The listing builds one solid part. Answer for the finished solid, in the listing's coordinates (mm). A direction names the side the tool comes from. Give positions to 0.01 mm unless a question says otherwise; leave off trailing zeros. Order: outer loops, then holes, each group sorted by start corner. A loop starts at its lowest first (then second) coordinate and runs counter-clockwise, first axis right, second up.
```python
from build123d import *

# Parameters (mm, degrees)
BOSS_EXTRUDE1_DEPTH = 5
FILLET1_R           = 8
BOSS_EXTRUDE2_DEPTH = 35
CUT_EXTRUDE1_DEPTH  = 40
CUT_EXTRUDE2_DEPTH  = 5
SKETCH9_W           = 9.5
SKETCH9_H           = 40
BOSS_EXTRUDE3_DEPTH = 3
SKETCH10_R          = 1.6
SKETCH10_W          = 6
SKETCH10_H          = 10
CUT_EXTRUDE3_DEPTH  = 3
SKETCH11_W          = 9.5
SKETCH11_H          = 4
BOSS_EXTRUDE4_DEPTH = 40
SKETCH13_W          = 25
SKETCH13_H          = 5
BOSS_EXTRUDE5_DEPTH = 15
SKETCH15_R          = 1.6
CUT_EXTRUDE4_DEPTH  = 5
CUT_EXTRUDE5_DEPTH  = 5
SKETCH17_W          = 17
SKETCH17_H          = 5
BOSS_EXTRUDE6_DEPTH = 9
SKETCH18_R          = 1.6
CUT_EXTRUDE6_DEPTH  = 5
CUT_EXTRUDE8_DEPTH  = 5


with BuildPart() as part:
    # Sketch1 → Boss-Extrude1 (new body)
    with BuildSketch(Plane(origin=(0, 0, 0), x_dir=(1, 0, 0), z_dir=(0, 1, 0))):
        Polygon((-75.055534995, 0), (-37.527767497, -65), (37.527767497, -65), (75.055534995, 0), (37.527767497, 65), (-37.527767497, 65), align=None)
    extrude(amount=BOSS_EXTRUDE1_DEPTH)

    # Fillet1
    fillet1_edges = [part.edges().sort_by_distance(p)[0] for p in [
        (-37.527767497, 2.5, -65),
        (37.527767497, 2.5, -65),
        (75.055534995, 2.5, 0),
        (37.527767497, 2.5, 65),
        (-37.527767497, 2.5, 65),
        (-75.055534995, 2.5, 0),
    ]]
    fillet(fillet1_edges, radius=FILLET1_R)

    # Sketch3 → Boss-Extrude2 (add)
    with BuildSketch(Plane(origin=(0, 5, 0), x_dir=(1, 0, 0), z_dir=(0, 1, 0))):
        with BuildLine():
            Line((-25, 65), (25, 65))
            ThreePointArc((25, 65), (30.656854249, 62.656854249), (33, 57))
            Line((33, 57), (33, -57))
            ThreePointArc((33, -57), (30.656854249, -62.656854249), (25, -65))
            Line((25, -65), (-25, -65))
            ThreePointArc((-25, -65), (-30.656854249, -62.656854249), (-33, -57))
            Line((-33, -57), (-33, 57))
            ThreePointArc((-33, 57), (-30.656854249, 62.656854249), (-25, 65))
        make_face()
    extrude(amount=BOSS_EXTRUDE2_DEPTH)

    # Sketch4 → Cut-Extrude1 (cut)
    with BuildSketch(Plane(origin=(0, 40, 0), x_dir=(1, 0, 0), z_dir=(0, 1, 0))):
        Polygon((-28, 57), (-25, 60), (25, 60), (28, 57), (28, -57), (25, -60), (-25, -60), (-28, -57), align=None)
    extrude(amount=-CUT_EXTRUDE1_DEPTH, mode=Mode.SUBTRACT)

    # Sketch8 → Cut-Extrude2 (cut)
    with BuildSketch(Plane(origin=(0, 0, 0), x_dir=(1, 0, 0), z_dir=(0, 1, 0))):
        with BuildLine():
            Line((-37.866025404, 44.41412012), (-58.889727457, 8))
            ThreePointArc((-58.889727457, 8), (-58.889727457, 6), (-57.15767665, 5))
            Line((-57.15767665, 5), (-38, 5))
            ThreePointArc((-38, 5), (-36.585786438, 5.585786438), (-36, 7))
            Line((-36, 7), (-36, 43.91412012))
            ThreePointArc((-36, 43.91412012), (-36.741180955, 44.880045946), (-37.866025404, 44.41412012))
        make_face()
        with BuildLine():
            Line((-36, -7), (-36, -43.91412012))
            ThreePointArc((-36, -43.91412012), (-36.741180955, -44.880045946), (-37.866025404, -44.41412012))
            Line((-37.866025404, -44.41412012), (-58.889727457, -8))
            ThreePointArc((-58.889727457, -8), (-58.889727457, -6), (-57.15767665, -5))
            Line((-57.15767665, -5), (-38, -5))
            ThreePointArc((-38, -5), (-36.585786438, -5.585786438), (-36, -7))
        make_face()
        with BuildLine():
            Line((37.866025404, -44.41412012), (58.889727457, -8))
            ThreePointArc((58.889727457, -8), (58.889727457, -6), (57.15767665, -5))
            Line((57.15767665, -5), (38, -5))
            ThreePointArc((38, -5), (36.585786438, -5.585786438), (36, -7))
            Line((36, -7), (36, -43.91412012))
            ThreePointArc((36, -43.91412012), (36.741180955, -44.880045946), (37.866025404, -44.41412012))
        make_face()
        with BuildLine():
            Line((36, 7), (36, 43.91412012))
            ThreePointArc((36, 43.91412012), (36.741180955, 44.880045946), (37.866025404, 44.41412012))
            Line((37.866025404, 44.41412012), (58.889727457, 8))
            ThreePointArc((58.889727457, 8), (58.889727457, 6), (57.15767665, 5))
            Line((57.15767665, 5), (38, 5))
            ThreePointArc((38, 5), (36.585786438, 5.585786438), (36, 7))
        make_face()
    extrude(amount=CUT_EXTRUDE2_DEPTH, mode=Mode.SUBTRACT)

    # Sketch9 → Boss-Extrude3 (add)
    with BuildSketch(Plane.XZ):
        with Locations((23.25, 0.197193855)):
            Rectangle(SKETCH9_W, SKETCH9_H)
        with Locations((-23.25, 0.197193855)):
            Rectangle(SKETCH9_W, SKETCH9_H)
    extrude(amount=-BOSS_EXTRUDE3_DEPTH)

    # Sketch10 → Cut-Extrude3 (cut)
    with BuildSketch(Plane(origin=(0, 3, 0), x_dir=(1, 0, 0), z_dir=(0, 1, 0))):
        with Locations(Location((23.25, -15.197193855, 0), (0, 0, 270))):
            Circle(SKETCH10_R)
        with Locations(Location((23.25, 14.802806145, 0), (0, 0, 270))):
            Circle(SKETCH10_R)
        with Locations(Location((-23.25, 14.802806145, 0), (0, 0, 270))):
            Circle(SKETCH10_R)
        with Locations(Location((-23.25, -15.197193855, 0), (0, 0, 270))):
            Circle(SKETCH10_R)
        with Locations((23.25, -0.197193855)):
            Rectangle(SKETCH10_W, SKETCH10_H)
        with Locations((-23.25, -0.197193855)):
            Rectangle(SKETCH10_W, SKETCH10_H)
    extrude(amount=-CUT_EXTRUDE3_DEPTH, mode=Mode.SUBTRACT)

    # Sketch11 → Boss-Extrude4 (add)
    with BuildSketch(Plane.XZ):
        with Locations((-23.25, 25.399999855)):
            Rectangle(SKETCH11_W, SKETCH11_H)
        Polygon((-28, 20.197193855), (-28, 21.197193855), (-18.5, 21.197193855), (-18.5, 18.394387855), (-28, 18.394387855), align=None)
        with Locations((23.25, 25.399999855)):
            Rectangle(SKETCH11_W, SKETCH11_H)
        Polygon((18.5, 21.197193855), (28, 21.197193855), (28, 20.197193855), (28, 18.394387855), (18.5, 18.394387855), align=None)
    extrude(amount=-BOSS_EXTRUDE4_DEPTH)

    # Sketch13 → Boss-Extrude5 (add)
    with BuildSketch(Plane(origin=(0, 0, 60), x_dir=(-1, 0, 0), z_dir=(0, 0, -1))):
        with Locations((0, 2.5)):
            Rectangle(SKETCH13_W, SKETCH13_H)
    extrude(amount=BOSS_EXTRUDE5_DEPTH)

    # Sketch15 → Cut-Extrude4 (cut)
    with BuildSketch(Plane.XZ):
        with Locations(Location((3.25, 48.75, 0), (0, 0, 270))):
            Circle(SKETCH15_R)
        with Locations(Location((3.25, 56.25, 0), (0, 0, 270))):
            Circle(SKETCH15_R)
        with Locations(Location((-3.25, 48.75, 0), (0, 0, 270))):
            Circle(SKETCH15_R)
        with Locations(Location((-3.25, 56.25, 0), (0, 0, 270))):
            Circle(SKETCH15_R)
    extrude(amount=-CUT_EXTRUDE4_DEPTH, mode=Mode.SUBTRACT)

    # Sketch16 → Cut-Extrude5 (cut)
    with BuildSketch(Plane.XY.offset(65)):
        Polygon((-12.75, 5), (12.75, 5), (12.75, 8.4), (8.75, 8.4), (8.75, 26.25), (-8.75, 26.25), (-8.75, 8.4), (-12.75, 8.4), align=None)
    extrude(amount=-CUT_EXTRUDE5_DEPTH, mode=Mode.SUBTRACT)

    # Sketch17 → Boss-Extrude6 (add)
    with BuildSketch(Plane.XY.offset(-60)):
        with Locations((0, 2.5)):
            Rectangle(SKETCH17_W, SKETCH17_H)
    extrude(amount=BOSS_EXTRUDE6_DEPTH)

    # Sketch18 → Cut-Extrude6 (cut)
    with BuildSketch(Plane.XZ):
        with Locations(Location((-3.25, -54.75, 0), (0, 0, 270))):
            Circle(SKETCH18_R)
        with Locations(Location((3.25, -54.75, 0), (0, 0, 90))):
            Circle(SKETCH18_R)
    extrude(amount=-CUT_EXTRUDE6_DEPTH, mode=Mode.SUBTRACT)

    # Sketch19 → Cut-Extrude8 (cut)
    with BuildSketch(Plane(origin=(0, 0, -65), x_dir=(-1, 0, 0), z_dir=(0, 0, -1))):
        Polygon((0, 5), (-8.75, 5), (-8.75, 26.4), (8.75, 26.4), (8.75, 5), align=None)
    extrude(amount=-CUT_EXTRUDE8_DEPTH, mode=Mode.SUBTRACT)


solid = part.part
```
1) Given P1, Ø9, axis at y = 14.5, z = 35, coming from the +X side; P2, Ø5.5, axis at x = 45.5, y = 3.5, coming from the -Z side; P3, Ø10, axis at y = 29, z = -47, coming from the -X side; P4, Ø22, axis at x = -4.5, z = 58, coming from the +Y side, each flat-ended and moving along its own axis, determine where each tip first touches the part or whether it passes through.
Geometry says:
P1: stops at x = 33
P2: stops at z = -55.95
P3: stops at x = -33
P4: stops at y = 40
2) A tool of negligible diameter and unlimited length cuts with its end or side. For faces 1 (the cylindrical face through (-30.719, 22.255, -62.594)), 2 (the flat face through (12.75, 7, 63)), 3 (the flat face through (-36, 2, 25)), from which of +Z, -Z, +X, -X, +Y, -Y can it reach the whole face along a straight path? Write none if from no direction.
Geometry says:
face 1: -Z, -X, +Y
face 2: +Z
face 3: +Y, -Y
3) For a pull along X with two mould halves and no side action, classify faces 4 (the flat face through (-8.75, 16, -63)), 5 (the cylindrical face through (-73.818, 2.535, 0.059)), 6 (the flat face through (-19, 40, 20)) as +X half, -X half, draft (parallel to the pull), parting line (faces both ways), or undercut.
Geometry says:
face 4: undercut
face 5: -X half
face 6: draft
4) Find section B-B (x = 16.5). Write down the section's boundary in (y, z), then the cut area to 3 significant figures.
Geometry says:
outline: (0, -65) - (40, -65) - (40, -60) - (0, -60) - close; (0, 60) - (40, 60) - (40, 65) - (0, 65) - close
area: 400 mm2
5) Find section D-D (z = -47.5). Write down the section's boundary in (x, y), then the cut area to 3 significant figures.
Geometry says:
outline: (-47.63, 0) - (-28, 0) - (-28, 40) - (-33, 40) - (-33, 5) - (-47.63, 5) - close; (28, 0) - (47.63, 0) - (47.63, 5) - (33, 5) - (33, 40) - (28, 40) - close
area: 546 mm2
6) Find section C-C (z = -29.5). Write down the section's boundary in (x, y), then the cut area to 3 significant figures.
Geometry says:
outline: (-58.02, 0) - (-46.48, 0) - (-46.48, 5) - (-58.02, 5) - close; (-36, 0) - (-28, 0) - (-28, 40) - (-33, 40) - (-33, 5) - (-36, 5) - close; (28, 0) - (36, 0) - (36, 5) - (33, 5) - (33, 40) - (28, 40) - close; (46.48, 0) - (58.02, 0) - (58.02, 5) - (46.48, 5) - close
area: 545 mm2
7) Straight lines are drawn through the part: probe 1 along Z at (x, y) = (-3, 1); probe 2 along Z at (x, y) = (-22, 20); probe 3 along X at (y, z) = (15, -46.5). For each, find the intervals that lie inside material, in ascending order.
Geometry says:
probe 1: z = -65 to -56.33, -53.17 to -51, 45 to 47.17, 50.33 to 54.67, 57.83 to 65
probe 2: z = -65 to -60, 18.39 to 21.2, 23.4 to 27.4, 60 to 65
probe 3: x = -33 to -28, 28 to 33
